Could you check a few things on this model? Use its own coordinates, in mm. Give positions to 0.01 mm unless a question says otherwise; leave off trailing zeros. Order: outer loops, then holes, each group sorted by start corner. A loop starts at its lowest first (then second) coordinate and runs counter-clockwise, first axis right, second up. Notation, with made-up numbers: (-33.75, 38.5) - (-15.75, 38.5) arc R25 cw to (-15.75, 55.5) - close; hole circle Ø1 at (56, 87). An arc over 180 degrees is marked (long way). One line per question, with ' | ' between items. Start each with the question number.
1. Imagine slicing it at C-C (y = -0.8). Please give me the cut outline in (x, z).
2. If we mould it in two halves opening along Z, with no side actions, what happens to faces 1 (the cylindrical face through (24.16, -1.01, 36.69)), 2 (the flat face through (0, -1, 35)), 3 (the cylindrical face through (39.24, -1.014, 16.983)), 4 (the flat face through (26, -1, 70))? For each: released by +Z, released by -Z, zero draft, split by the parting line, or undercut.
3. For P1, Ø1, axis at y = -1, z = 48.5, coming from the +X side; P2, Ø8, axis at x = 26, z = 60, coming from the -Y side, each with a flat end and sliding along its axis, tell me the tip position at first contact or that it passes through.
4. I need wall thicknesses on probe 1 along Z at (x, y) = (26, -0.75); probe 2 along Z at (x, y) = (12.5, -0.7); probe 3 along X at (y, z) = (-1.7, 13.5). Which ranges of each line are inside material? Lowest first, please. Write a range as from..to.
5. Imagine slicing it at A-A (x = 26). Please give me the cut outline in (y, z), and give its area (3 significant figures).
6. Imagine slicing it at D-D (z = 15). Give the number of separate pieces and of enclosed holes in the cut face, and give its area (3 significant figures).
```python
from build123d import *

# Parameters (mm, degrees)
F0_W     = 50
F0_H     = 70
F1_DEPTH = 2
F2_R     = 1.99999
F3_R     = 2
F3_R_2   = 2.5
F4_DEPTH = 2.001


# Not quite as in the source:
# - a fillet or chamfer is up to 0.001 mm smaller than in the source, because OpenCascade refuses the exact size


with BuildPart() as f1:
    # F0 (on Front) → F1 (new body)
    with BuildSketch(Plane.XZ):
        with Locations((25, 35)):
            Rectangle(F0_W, F0_H)
    extrude(amount=F1_DEPTH)

    # F2 (radius 2 in the source; OpenCascade refuses exactly that, so slightly less here)
    f2_edges = [f1.edges().sort_by_distance(p)[0] for p in [
        (0, -1, 0),
        (50, -1, 0),
        (50, 0, 35),
        (0, -1, 70),
    ]]
    fillet(f2_edges, radius=F2_R)

    # F3 (on face) → F4 (cut, through all)
    with BuildSketch(Plane.XZ.offset(2)):
        with Locations((12.5, 15)):
            Circle(F3_R)
        with Locations((39.5, 15)):
            Circle(F3_R)
        with Locations((26, 60)):
            Circle(F3_R_2)
        with Locations((26, 35)):
            Circle(F3_R_2)
    extrude(amount=-F4_DEPTH, mode=Mode.SUBTRACT)


solid = f1.part
```
Results found:
1) outline: (0, 2) arc R2 ccw to (2, 0) - (48, 0) arc R2 ccw to (49.6, 0.8) - (49.6, 70) - (2, 70) arc R2 ccw to (0, 68) - close; hole circle Ø4 at (12.5, 15); hole circle Ø5 at (26, 35); hole circle Ø5 at (26, 60); hole circle Ø4 at (39.5, 15)
2) face 1: undercut | face 2: zero draft | face 3: undercut | face 4: released by +Z
3) P1: stops at x = 49.94 | P2: stops at y = -2
4) probe 1: z = 0..32.5, 37.5..57.5, 62.5..70 | probe 2: z = 0..13, 17..70 | probe 3: x = 0..11.18, 13.82..38.18, 40.82..49.98
5) outline: (-2, 0) - (0, 0) - (0, 32.5) - (-2, 32.5) - close; (-2, 37.5) - (0, 37.5) - (0, 57.5) - (-2, 57.5) - close; (-2, 62.5) - (0, 62.5) - (0, 70) - (-2, 70) - close | area: 120 mm2
6) separate pieces: 3 | enclosed holes: 0 | area: 83.1 mm2
